from build123d import *

# Parameters (mm, degrees)
F0_R     = 13.3987059817
F1_DEPTH = 64.516
F3_R     = 14.8099324152
F4_DEPTH = 61.976


with BuildPart() as f1:
    # F0 (on Top) → F1 (new body)
    with BuildSketch(Plane.XY):
        Circle(F0_R)
    extrude(amount=F1_DEPTH)


with BuildPart() as f4:
    # F3 (on Right) → F4 (new body)
    with BuildSketch(Plane.YZ):
        with Locations((-0.4007364958, 1.1823429543)):
            Circle(F3_R)
    extrude(amount=F4_DEPTH)


solid = f4.part
Input: part model. Units: mm. Frame: model coordinates. Round coordinates to 2 decimals unless told otherwise and drop trailing zeros. Order: outer loops, then holes, each group sorted by start corner. A loop starts at its lowest first (then second) coordinate and runs counter-clockwise, first axis right, second up. Notation, with made-up numbers: (36, -14) - (62, -14) arc R27 cw to (62, 19) - close; hole circle Ø7 at (19, 40.25). An arc over 180 degrees is marked (long way). Use a Markdown table: item, result.
1. Material intervals for probe 1 along Z at (x, y) = (21.5, -1); probe 2 along Z at (x, y) = (18, -7.5); probe 3 along Y at (x, z) = (16, -2.5), sorted ascending.
Evaluation:
| item | result |
|---|---|
| probe 1 | -13.62 to 15.98 |
| probe 2 | -11.82 to 14.18 |
| probe 3 | -14.75 to 13.94 |
2. Section C-C on x = 32. Return the cut outline in (y, z).
Evaluation:
| item | result |
|---|---|
| outline | circle Ø29.62 at (-0.4, 1.18) |
3. Section A-A on z = -8.25. Return the cut outline in (x, y).
Evaluation:
| item | result |
|---|---|
| outline | (0, -11.82) - (61.98, -11.82) - (61.98, 11.02) - (0, 11.02) - close |
4. First-contact query: pin 1 (2 mm diameter, centred on x = 6.5, y = -4.5, fed in from -Z); pin 2 (12 mm diameter, centred on x = 19, z = -5, fed in from +Y); pin 3 (1.5 mm diameter, centred on x = 46, y = 5.5, fed in from -Z). Flat tips, straight axial feed; report the tip coordinate or a pass-through.
Evaluation:
| item | result |
|---|---|
| pin 1 | z = -13.3 |
| pin 2 | y = 14.41 |
| pin 3 | z = -12.7 |
5. Section B-B on y = 4.5. Return the cut outline in (x, z), then the cut area to 3 significant figures.
Evaluation:
| item | result |
|---|---|
| outline | (0, -12.79) - (61.98, -12.79) - (61.98, 15.16) - (0, 15.16) - close |
| area | 1,730 mm^2 |
